Design review of the part built by this model. Coordinates are the model's own, in mm. Give positions to 0.01 mm unless a question says otherwise; leave off trailing zeros. Loops run counter-clockwise (first coordinate to the right, second up) from the corner with the lowest first, then second, coordinate; pieces in that order, holes last. Notation, with made-up numbers: (72.25, -2.5) -> (122.25, -2.5) arc R9 ccw to (122.25, 2.5) -> close; hole circle Ø10 at (31, -37). An arc over 180 degrees is marked (long way). Answer in a Markdown table with one row per item. Add a question column.
(1) Consider section D-D on y = 7.25. Count the separate pieces of the cut face and the enclosed holes in it, then the cut area to 3 significant figures.
(2) Consider section B-B on x = 63. Write out the cut boundary in (y, z).
(3) Consider section A-A on z = -21. Write out the cut boundary in (x, y), then the cut area to 3 significant figures.
(4) Consider section C-C on z = 42. Write out the cut boundary in (x, y), then the cut area to 3 significant figures.
(5) For line 1 (X direction, y = 5, z = 21); line 2 (Z direction, x = 42.5, y = 5.5); line 3 (X direction, y = 7, z = 42), list the stretches that pass through material, from the lowest coordinate up.
(6) For pin 1 (8 mm diameter, centred on x = 0, z = 42, fed in from +Y), flat-tipped, find the tip position at first contact; note if it passes through.
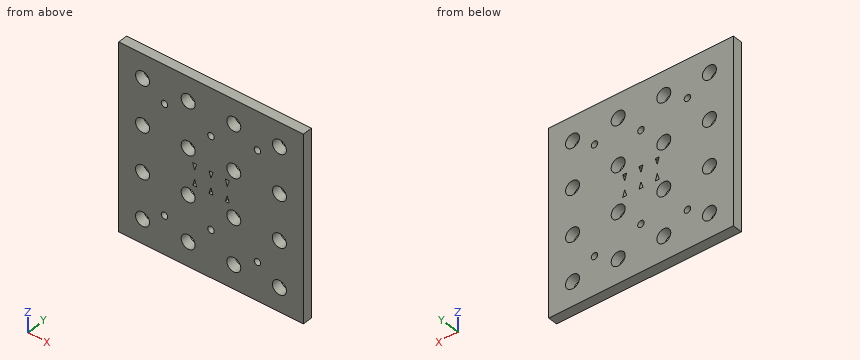
Autodesk Inventor part; units mm, degrees
ref_plane "YZ Plane" through (0, 0, 0) normal (1, 0, 0) x (0, 1, 0)
ref_plane "XZ Plane" through (0, 0, 0) normal (0, 1, 0) x (-1, 0, 0)
ref_plane "XY Plane" through (0, 0, 0) normal (0, 0, 1) x (1, 0, 0)
sketch "Sketch1" plane through (0, 0, 0) normal (0, 1, 0) x (-1, 0, 0)
  line L0 (-85, 85) -> (85, 85)
  line L1 (85, 85) -> (85, -85)
  line L2 (85, -85) -> (-85, -85)
  line L3 (-85, -85) -> (-85, 85)
  line L4 (-85, 85) -> (85, -85) construction
  line L5 (85, 85) -> (-85, -85) construction
  point P0 (0, 0)
  point P1 (-63, -63)
  point P2 (-63, -21)
  point P3 (-63, 21)
  point P4 (-63, 63)
  point P5 (-21, -63)
  point P6 (-21, -21)
  point P7 (-21, 21)
  point P8 (-21, 63)
  point P9 (21, -63)
  point P10 (21, -21)
  point P11 (21, 21)
  point P12 (21, 63)
  point P13 (63, -63)
  point P14 (63, -21)
  point P15 (63, 21)
  point P16 (63, 63)
  dimension "d0" = 170
  dimension "d1" = 170
  dimension "d4" = 42
  dimension "d7" = 42
extrude "Extrusion1" add sketch "Sketch1" along normal blind 9
hole "Hole1" at (63, 0, -63) at (63, 0, -21) at (63, 0, 21) at (63, 0, 63) at (21, 0, -63) at (21, 0, -21) at (21, 0, 21) at (21, 0, 63) at (-21, 0, -63) at (-21, 0, -21) at (-21, 0, 21) at (-21, 0, 63) at (-63, 0, -63) at (-63, 0, -21) at (-63, 0, 21) at (-63, 0, 63) direction (0, 1, 0) diameter 12.86 end through all both
sketch "Sketch2" plane through (0, 9, 0) normal (0, 1, 0) x (1, 0, 0)
  line L0 (-33.7, -4.15) -> (33.7, -4.15)
  line L1 (33.7, -4.15) -> (33.7, 4.15)
  line L2 (33.7, 4.15) -> (-33.7, 4.15)
  line L3 (-33.7, 4.15) -> (-33.7, -4.15)
  line L4 (-33.7, -4.15) -> (33.7, 4.15) construction
  line L5 (33.7, -4.15) -> (-33.7, 4.15) construction
  point P0 (0, 0)
  dimension "d19" = 67.4
  dimension "d20" = 8.3
sketch "Sketch3" plane through (0, 9, 0) normal (0, 1, 0) x (1, 0, 0)
  line L0 (-42.7949, -50) -> (42.7949, -50) construction
  line L1 (42.7949, -50) -> (42.7949, 50) construction
  line L2 (42.7949, 50) -> (-42.7949, 50) construction
  line L3 (-42.7949, 50) -> (-42.7949, -50) construction
  line L4 (-42.7949, -50) -> (42.7949, 50) construction
  line L5 (42.7949, -50) -> (-42.7949, 50) construction
  point P0 (25, -42.5)
  point P1 (0, 0)
  dimension "d31" = 100
hole "Hole3" at (-42.7949, 9, -50) at (42.7949, 9, -50) at (42.7949, 9, 50) at (-42.7949, 9, 50) direction (0, -1, 0) diameter 6 end through all both
sketch "Sketch4" plane through (0, 9, 0) normal (0, 1, 0) x (1, 0, 0)
  circle A0 centre (42.7949, -50) radius 3 construction
  circle A1 centre (-42.7949, 50) radius 3 construction
  circle A2 centre (42.7949, 50) radius 3 construction
  circle A3 centre (-42.7949, -50) radius 3 construction
  circle A4 centre (-63, -21) radius 6.43 construction
  circle A5 centre (-63, 63) radius 6.43 construction
  circle A6 centre (-21, -21) radius 6.43 construction
  circle A7 centre (-21, 63) radius 6.43 construction
  circle A8 centre (21, -21) radius 6.43 construction
  circle A9 centre (21, 63) radius 6.43 construction
  circle A10 centre (63, -21) radius 6.43 construction
  circle A11 centre (63, 63) radius 6.43 construction
  circle A12 centre (63, 21) radius 6.43 construction
  circle A13 centre (63, -63) radius 6.43 construction
  circle A14 centre (21, 21) radius 6.43 construction
  circle A15 centre (21, -63) radius 6.43 construction
  circle A16 centre (-21, 21) radius 6.43 construction
  circle A17 centre (-21, -63) radius 6.43 construction
  circle A18 centre (-63, 21) radius 6.43 construction
  circle A19 centre (-63, -63) radius 6.43 construction
  line L0 (-85, -85) -> (85, -85) construction
  line L1 (85, -85) -> (85, 85) construction
  line L2 (85, 85) -> (-85, 85) construction
  line L3 (-85, 85) -> (-85, -85) construction
  line L4 (-85, 85) -> (85, 85) construction
  line L5 (-7.5, -85) -> (7.5, -85) construction
  line L6 (7.5, -85) -> (7.5, 85) construction
  line L7 (7.5, 85) -> (-7.5, 85) construction
  line L8 (-7.5, 85) -> (-7.5, -85) construction
  line L9 (-7.5, -85) -> (7.5, 85) construction
  line L10 (7.5, -85) -> (-7.5, 85) construction
  line L11 (-21, 63) -> (21, 63) construction
  line L12 (21, 63) -> (21, 21) construction
  line L13 (21, 21) -> (-21, 21) construction
  line L14 (-21, 21) -> (-21, 63) construction
  line L15 (-85, 0) -> (85, 0) construction
  point P0 (0, 0)
  point P1 (0, 42)
  point P2 (0, -42)
  dimension "d39" = 15
hole "Hole4" at (0, 9, -42) at (0, 9, 42) direction (0, -1, 0) diameter 6 end through all both
sketch "Sketch5" plane through (0, 9, 0) normal (0, 1, 0) x (1, 0, 0)
  line L0 (-33.7, -10) -> (33.7, -10) construction
  line L1 (33.7, -10) -> (33.7, 10) construction
  line L2 (33.7, 10) -> (-33.7, 10) construction
  line L3 (-33.7, 10) -> (-33.7, -10) construction
  line L4 (-33.7, -10) -> (33.7, 10) construction
  line L5 (33.7, -10) -> (-33.7, 10) construction
  line L6 (0, 10) -> (0, -10) construction
  line L7 (-1.8038, 10) -> (0, 4.1128)
  line L8 (1.8038, 10) -> (0, 4.1128)
  line L9 (-1.8038, 10) -> (1.8038, 10)
  line L10 (-33.7, 0) -> (33.7, 0) construction
  line L11 (-1.8038, -10) -> (0, -4.1128)
  line L12 (1.8038, -10) -> (0, -4.1128)
  line L13 (-1.8038, -10) -> (1.8038, -10)
  line L14 (-16.8038, 10) -> (-15, 4.1128)
  line L15 (-13.1962, 10) -> (-15, 4.1128)
  line L16 (-16.8038, 10) -> (-13.1962, 10)
  line L17 (13.1962, 10) -> (15, 4.1128)
  line L18 (16.8038, 10) -> (15, 4.1128)
  line L19 (13.1962, 10) -> (16.8038, 10)
  line L20 (-1.8038, 10) -> (0, 4.1128)
  line L21 (1.8038, 10) -> (0, 4.1128)
  line L22 (-1.8038, 10) -> (1.8038, 10)
  line L23 (-16.8038, -10) -> (-15, -4.1128)
  line L24 (-13.1962, -10) -> (-15, -4.1128)
  line L25 (-16.8038, -10) -> (-13.1962, -10)
  line L26 (13.1962, -10) -> (15, -4.1128)
  line L27 (16.8038, -10) -> (15, -4.1128)
  line L28 (13.1962, -10) -> (16.8038, -10)
  point P0 (0, 0)
  point P1 (-15, 10)
  point P2 (15, 10)
  point P3 (-15, -10)
  point P4 (15, -10)
  dimension "d47" = 67.4
  dimension "d50" = 20
  dimension "d53" = 15
  dimension "d56" = 15
extrude "Extrusion2" cut sketch "Sketch5" against normal blind 10 contours L9 L8 L7 | L11 L12 L13
extrude "Extrusion3" cut sketch "Sketch5" against normal blind 10 contours L16 L15 L14 | L19 L18 L17 | L23 L24 L25 | L26 L27 L28
properties part number "front_plate"
Values follow:
| question | item | result |
|---|---|---|
| 1 | separate pieces | 1 |
| 1 | enclosed holes | 28 |
| 1 | area | 26,600 mm2 |
| 2 | outline | (0, -85) -> (9, -85) -> (9, -69.43) -> (0, -69.43) -> close; (0, -56.57) -> (9, -56.57) -> (9, -27.43) -> (0, -27.43) -> close; (0, -14.57) -> (9, -14.57) -> (9, 14.57) -> (0, 14.57) -> close; (0, 27.43) -> (9, 27.43) -> (9, 56.57) -> (0, 56.57) -> close; (0, 69.43) -> (9, 69.43) -> (9, 85) -> (0, 85) -> close |
| 3 | outline | (-85, 0) -> (-69.43, 0) -> (-69.43, 9) -> (-85, 9) -> close; (-56.57, 0) -> (-27.43, 0) -> (-27.43, 9) -> (-56.57, 9) -> close; (-14.57, 0) -> (14.57, 0) -> (14.57, 9) -> (-14.57, 9) -> close; (27.43, 0) -> (56.57, 0) -> (56.57, 9) -> (27.43, 9) -> close; (69.43, 0) -> (85, 0) -> (85, 9) -> (69.43, 9) -> close |
| 3 | area | 1,070 mm2 |
| 4 | outline | (-85, 0) -> (-3, 0) -> (-3, 9) -> (-85, 9) -> close; (3, 0) -> (85, 0) -> (85, 9) -> (3, 9) -> close |
| 4 | area | 1,480 mm2 |
| 5 | line 1 | -85 to -69.43, -56.57 to -27.43, -14.57 to 14.57, 27.43 to 56.57, 69.43 to 85 |
| 5 | line 2 | -85 to -52.99, -47.01 to 47.01, 52.99 to 85 |
| 5 | line 3 | -85 to -3, 3 to 85 |
| 6 | pin 1 | y = 9 |
